from build123d import *

# Parameters (mm, degrees)
SKETCH1_R           = 40
BOSS_EXTRUDE1_DEPTH = 40
SHELL1_T            = -1.45
FILLET1_R           = 5


with BuildPart() as part:
    # Sketch1 → Boss-Extrude1 (new body)
    with BuildSketch(Plane.XY):
        Circle(SKETCH1_R)
    extrude(amount=BOSS_EXTRUDE1_DEPTH)

    # Shell1
    shell1_openings = [part.faces().sort_by_distance(p)[0] for p in [
        (0, 0, 40),
    ]]
    offset(amount=SHELL1_T, openings=shell1_openings, kind=Kind.INTERSECTION)

    # Fillet1
    fillet1_edges = [part.edges().sort_by_distance(p)[0] for p in [
        (-40, 0, 0),
        (-38.55, 0, 1.45),
    ]]
    fillet(fillet1_edges, radius=FILLET1_R)


solid = part.part
Can you work these out from the model? Positions are in its coordinate system, mm. A direction names the side the tool comes from. Coordinates: 2 decimals unless noted, no trailing zeros. Write each loop counter-clockwise with the first axis right and the second up, starting at its lowest first coordinate (ties: lowest second). Pieces come first, ordered by that corner, then holes. Notation, with made-up numbers: (-31.75, -10.75) - (-18.75, -10.75) arc R21 cw to (-18.75, -1.75) - close; hole circle Ø11 at (3, -7). An arc over 180 degrees is marked (long way). Return JSON: item names as keys, results as strings. Group by question number.
Item 1: Which directions (+Z, -Z, +X, -X, +Y, -Y) give clear straight access to the entire face, cutting with the end or side of a thin tool? Please do faces 4 (the face through (-21, 33, 40)), 5 (the face through (0, 0, 1.45)).
Item 2: If we section it at B-B (z = 31.5): Write out the boundary of the cut face in (x, y).
Item 3: We'd pull the mould along Y, two halves only. Please class faces 1 (the face through (-8.67, -39.05, 22.26)), 2 (the face through (0, 0, 0)), 3 (the face through (36.77, 11.58, 22.99)): pulls with the +Y half, pulls with the -Y half, needs draft (parallel to the pull), parting line crosses it, or undercut.
Item 4: I'm going to push flat-ended pins straight in: pin 1 Ø20 at (x, y) = (4.5, -5.5) entering from +Z; pin 2 Ø1 at (x, z) = (-20, 17) entering from -Y; pin 3 Ø1.5 at (y, z) = (-16.5, 14.5) entering from -X. Where does each tip first touch, or does it pass through?
Item 5: Please list where these lines run through material, in increasing order: probe 1 along X at (y, z) = (-1, 9.5); probe 2 along Y at (x, z) = (0, 17); probe 3 along Y at (x, z) = (-13, 29).
Item 6: If we section it at A-A (x = 0): Write out the boundary of the cut face in (y, z), then the cut area to 3 significant figures.
Return value:
{
 "1": {"face 4": "+Z, +X, -X, +Y, -Y", "face 5": "+Z"},
 "2": {"outline": "circle Ø80 at (0, 0); hole circle Ø77.1 at (0, 0)"},
 "3": {"face 1": "parting line crosses it", "face 2": "needs draft", "face 3": "undercut"},
 "4": {"pin 1": "stops at z = 1.45", "pin 2": "stops at y = -34.92", "pin 3": "stops at x = -36.77"},
 "5": {"probe 1": "x = -39.99 to -38.54, 38.54 to 39.99", "probe 2": "y = -40 to -38.55, 38.55 to 40", "probe 3": "y = -37.83 to -36.29, 36.29 to 37.83"},
 "6": {"outline": "(-40, 5) arc R5 ccw to (-35, 0) - (35, 0) arc R5 ccw to (40, 5) - (40, 40) - (38.55, 40) - (38.55, 6.45) arc R5 cw to (33.55, 1.45) - (-33.55, 1.45) arc R5 cw to (-38.55, 6.45) - (-38.55, 40) - (-40, 40) - close", "area": "228 mm^2"}
}
